Read the model definition and answer for the solid it produces. Units are mm, in the model's axes. A direction names the side the tool comes from. Coordinates: 2 decimals unless noted, no trailing zeros. Write each loop counter-clockwise with the first axis right and the second up, starting at its lowest first coordinate (ties: lowest second). Pieces come first, ordered by that corner, then holes. Notation, with made-up numbers: (34, -26.75) -> (74, -26.75) arc R31 cw to (74, 3.25) -> close; hole circle Ø4 at (53, 39.5). An arc over 180 degrees is marked (long way). One line per item, written item: value. Start each with the question number.
1. Consider line 1 along Y through (x, z) = (0, 84); line 2 along Y through (x, z) = (0, -73); line 3 along Z through (x, y) = (-60, 67). Determine where each line is inside the solid, lowest interval first.
2. Find section A-A, the plane z = 72. State how many separate pieces and enclosed holes the cut face has, and give its area (3 significant figures).
3. For a pull along Z with two mould halves and no side action, classify faces 1 (the flat face through (-22.57, 50.35, -89)), 2 (the flat face through (-25, 21, -59)), 3 (the cylindrical face through (20.59, -92.74, -79.14)) as pulls with the +Z half, pulls with the -Z half, needs draft (parallel to the pull), parting line crosses it, or undercut.
4. Find section D-D, the plane y = -83.5. Write down the section's boundary in (x, z).
5. Given P1, Ø3, axis at x = 26.5, y = 27, coming from the +Z side; P2, Ø1, axis at x = -23, y = 46.5, coming from the -Z side; P3, Ø2, axis at x = -11.5, z = -52, coming from the +Y side, each flat-ended and moving along its own axis, determine where each tip first touches the part or whether it passes through.
6. Find section B-B, the plane z = -77. Write down the section's boundary in (x, y).
7. For faces 4 (the cylindrical face through (9.764, 74.362, -79.14)), 5 (the flat face through (-24, -93, -89)), 6 (the flat face through (-1, -65, 1)), 7 (the cylindrical face through (48.627, 22.202, 68.126)), determine the directions among +Z, -Z, +X, -X, +Y, -Y from which every point of the face is accessible in a straight line to the end or side of a thin tool.
```python
from build123d import *

# Parameters (mm, degrees)
SKETCH_1_R           = 105
EXTRUDE_1_DEPTH      = 89
CUT_EXTRUDE_1_DEPTH  = 59
SKETCH_4_R           = 95
SKETCH_4_R_2         = 75
CUT_EXTRUDE_2_DEPTH  = 20
SKETCH_5_R           = 55
CUT_EXTRUDE_3_DEPTH  = 22
SKETCH_6_R           = 50
CUT_EXTRUDE_4_DEPTH  = 3
CUT_EXTRUDE_5_REACH  = 215.211
SKETCH_7_R           = 31
CUT_EXTRUDE_START    = -20
SKETCH_8_R           = 95
SKETCH_8_R_2         = 75
CUT_EXTRUDE_6_DEPTH  = 20
SKETCH_9_R           = 67.5
CUT_EXTRUDE_7_DEPTH  = 12
CUT_EXTRUDE_8_REACH  = 224.724
SKETCH_10_R          = 32.5
CHAMFER_1_SIZE       = 2
CUT_EXTRUDE_9_REACH  = 218.827
SKETCH_11_R          = 5
CUT_EXTRUDE_10_REACH = 224.724
SKETCH_12_R          = 4.5


with BuildPart() as part:
    # 草图1 → 凸台-拉伸1 (new, symmetric)
    with BuildSketch(Plane.XY):
        Circle(SKETCH_1_R)
    extrude(amount=EXTRUDE_1_DEPTH, both=True)

    # 草图3 → 切除-拉伸1 (cut, symmetric)
    with BuildSketch(Plane.XY):
        with BuildLine():
            Line((-82.462112512, -65), (82.462112512, -65))
            ThreePointArc((82.462112512, -65), (0, 105), (-82.462112512, -65))
        make_face()
    extrude(amount=CUT_EXTRUDE_1_DEPTH, both=True, mode=Mode.SUBTRACT)

    # 草图4 → 切除-拉伸2 (cut)
    with BuildSketch(Plane(origin=(0, 0, -89), x_dir=(-1, 0, 0), z_dir=(0, 0, -1))):
        Circle(SKETCH_4_R)
        Circle(SKETCH_4_R_2, mode=Mode.SUBTRACT)
    extrude(amount=-CUT_EXTRUDE_2_DEPTH, mode=Mode.SUBTRACT)

    # 草图5 → 切除-拉伸3 (cut)
    with BuildSketch(Plane(origin=(0, 0, -89), x_dir=(-1, 0, 0), z_dir=(0, 0, -1))):
        Circle(SKETCH_5_R)
    extrude(amount=-CUT_EXTRUDE_3_DEPTH, mode=Mode.SUBTRACT)

    # 草图6 → 切除-拉伸4 (cut)
    with BuildSketch(Plane(origin=(0, 0, -67), x_dir=(-1, 0, 0), z_dir=(0, 0, -1))):
        Circle(SKETCH_6_R)
    extrude(amount=-CUT_EXTRUDE_4_DEPTH, mode=Mode.SUBTRACT)

    # 草图7 → 切除-拉伸5 (cut, up to next)
    with BuildSketch(Plane(origin=(0, 0, -64), x_dir=(-1, 0, 0), z_dir=(0, 0, -1)), mode=Mode.PRIVATE) as cut_extrude_5_sk1:
        Circle(SKETCH_7_R)
    cut_extrude_5_tool1 = extrude(cut_extrude_5_sk1.sketch, amount=-CUT_EXTRUDE_5_REACH, mode=Mode.PRIVATE) & part.part
    add(cut_extrude_5_tool1.solids().sort_by_distance((0, 0, -64))[0], mode=Mode.SUBTRACT)

    # 草图8 → 切除-拉伸6 (cut)
    with BuildSketch(Plane.XY.offset(89).offset(CUT_EXTRUDE_START)):
        with Locations(Location((0, 0, 0), (0, 0, 180))):
            Circle(SKETCH_8_R)
        with Locations(Location((0, 0, 0), (0, 0, 180))):
            Circle(SKETCH_8_R_2, mode=Mode.SUBTRACT)
    extrude(amount=CUT_EXTRUDE_6_DEPTH, mode=Mode.SUBTRACT)

    # 草图9 → 切除-拉伸7 (cut)
    with BuildSketch(Plane.XY.offset(89)):
        Circle(SKETCH_9_R)
    extrude(amount=-CUT_EXTRUDE_7_DEPTH, mode=Mode.SUBTRACT)

    # 草图10 → 切除-拉伸8 (cut, up to next)
    with BuildSketch(Plane.XY.offset(77), mode=Mode.PRIVATE) as cut_extrude_8_sk1:
        Circle(SKETCH_10_R)
    cut_extrude_8_tool1 = extrude(cut_extrude_8_sk1.sketch, amount=-CUT_EXTRUDE_8_REACH, mode=Mode.PRIVATE) & part.part
    add(cut_extrude_8_tool1.solids().sort_by_distance((0, 0, 77))[0], mode=Mode.SUBTRACT)

    # 倒角1
    chamfer_1_edges = [part.edges().sort_by_distance(p)[0] for p in [
        (-32.5, 0, 77),
    ]]
    chamfer(chamfer_1_edges, length=CHAMFER_1_SIZE)

    # 草图11 → 切除-拉伸9 (cut, up to next)
    with BuildSketch(Plane.XY.offset(69), mode=Mode.PRIVATE) as cut_extrude_9_sk1:
        with Locations((0, 85)):
            Circle(SKETCH_11_R)
    cut_extrude_9_tool1 = extrude(cut_extrude_9_sk1.sketch, amount=-CUT_EXTRUDE_9_REACH, mode=Mode.PRIVATE) & part.part
    # 草图11 → 切除-拉伸9 (cut, up to next)
    with BuildSketch(Plane.XY.offset(69), mode=Mode.PRIVATE) as cut_extrude_9_sk2:
        with Locations((32.528091751, 78.529760263)):
            Circle(SKETCH_11_R)
    cut_extrude_9_tool2 = extrude(cut_extrude_9_sk2.sketch, amount=-CUT_EXTRUDE_9_REACH, mode=Mode.PRIVATE) & part.part
    # 草图11 → 切除-拉伸9 (cut, up to next)
    with BuildSketch(Plane.XY.offset(69), mode=Mode.PRIVATE) as cut_extrude_9_sk3:
        with Locations((-32.528091751, 78.529760263)):
            Circle(SKETCH_11_R)
    cut_extrude_9_tool3 = extrude(cut_extrude_9_sk3.sketch, amount=-CUT_EXTRUDE_9_REACH, mode=Mode.PRIVATE) & part.part
    add(cut_extrude_9_tool1.solids().sort_by_distance((0, 85, 69))[0], mode=Mode.SUBTRACT)
    add(cut_extrude_9_tool2.solids().sort_by_distance((32.528092, 78.52976, 69))[0], mode=Mode.SUBTRACT)
    add(cut_extrude_9_tool3.solids().sort_by_distance((-32.528092, 78.52976, 69))[0], mode=Mode.SUBTRACT)

    # 草图12 → 切除-拉伸10 (cut, up to next)
    with BuildSketch(Plane.XY.offset(77), mode=Mode.PRIVATE) as cut_extrude_10_sk1:
        with Locations((22.004297361, 53.123073119)):
            Circle(SKETCH_12_R)
    cut_extrude_10_tool1 = extrude(cut_extrude_10_sk1.sketch, amount=-CUT_EXTRUDE_10_REACH, mode=Mode.PRIVATE) & part.part
    # 草图12 → 切除-拉伸10 (cut, up to next)
    with BuildSketch(Plane.XY.offset(77), mode=Mode.PRIVATE) as cut_extrude_10_sk2:
        with Locations((53.123073119, 22.004297361)):
            Circle(SKETCH_12_R)
    cut_extrude_10_tool2 = extrude(cut_extrude_10_sk2.sketch, amount=-CUT_EXTRUDE_10_REACH, mode=Mode.PRIVATE) & part.part
    # 草图12 → 切除-拉伸10 (cut, up to next)
    with BuildSketch(Plane.XY.offset(77), mode=Mode.PRIVATE) as cut_extrude_10_sk3:
        with Locations((53.123073119, -22.004297361)):
            Circle(SKETCH_12_R)
    cut_extrude_10_tool3 = extrude(cut_extrude_10_sk3.sketch, amount=-CUT_EXTRUDE_10_REACH, mode=Mode.PRIVATE) & part.part
    # 草图12 → 切除-拉伸10 (cut, up to next)
    with BuildSketch(Plane.XY.offset(77), mode=Mode.PRIVATE) as cut_extrude_10_sk4:
        with Locations((22.004297361, -53.123073119)):
            Circle(SKETCH_12_R)
    cut_extrude_10_tool4 = extrude(cut_extrude_10_sk4.sketch, amount=-CUT_EXTRUDE_10_REACH, mode=Mode.PRIVATE) & part.part
    # 草图12 → 切除-拉伸10 (cut, up to next)
    with BuildSketch(Plane.XY.offset(77), mode=Mode.PRIVATE) as cut_extrude_10_sk5:
        with Locations((-22.004297361, -53.123073119)):
            Circle(SKETCH_12_R)
    cut_extrude_10_tool5 = extrude(cut_extrude_10_sk5.sketch, amount=-CUT_EXTRUDE_10_REACH, mode=Mode.PRIVATE) & part.part
    # 草图12 → 切除-拉伸10 (cut, up to next)
    with BuildSketch(Plane.XY.offset(77), mode=Mode.PRIVATE) as cut_extrude_10_sk6:
        with Locations((-53.123073119, -22.004297361)):
            Circle(SKETCH_12_R)
    cut_extrude_10_tool6 = extrude(cut_extrude_10_sk6.sketch, amount=-CUT_EXTRUDE_10_REACH, mode=Mode.PRIVATE) & part.part
    # 草图12 → 切除-拉伸10 (cut, up to next)
    with BuildSketch(Plane.XY.offset(77), mode=Mode.PRIVATE) as cut_extrude_10_sk7:
        with Locations((-53.123073119, 22.004297361)):
            Circle(SKETCH_12_R)
    cut_extrude_10_tool7 = extrude(cut_extrude_10_sk7.sketch, amount=-CUT_EXTRUDE_10_REACH, mode=Mode.PRIVATE) & part.part
    # 草图12 → 切除-拉伸10 (cut, up to next)
    with BuildSketch(Plane.XY.offset(77), mode=Mode.PRIVATE) as cut_extrude_10_sk8:
        with Locations((-22.004297361, 53.123073119)):
            Circle(SKETCH_12_R)
    cut_extrude_10_tool8 = extrude(cut_extrude_10_sk8.sketch, amount=-CUT_EXTRUDE_10_REACH, mode=Mode.PRIVATE) & part.part
    add(cut_extrude_10_tool1.solids().sort_by_distance((22.004297, 53.123073, 77))[0], mode=Mode.SUBTRACT)
    add(cut_extrude_10_tool2.solids().sort_by_distance((53.123073, 22.004297, 77))[0], mode=Mode.SUBTRACT)
    add(cut_extrude_10_tool3.solids().sort_by_distance((53.123073, -22.004297, 77))[0], mode=Mode.SUBTRACT)
    add(cut_extrude_10_tool4.solids().sort_by_distance((22.004297, -53.123073, 77))[0], mode=Mode.SUBTRACT)
    add(cut_extrude_10_tool5.solids().sort_by_distance((-22.004297, -53.123073, 77))[0], mode=Mode.SUBTRACT)
    add(cut_extrude_10_tool6.solids().sort_by_distance((-53.123073, -22.004297, 77))[0], mode=Mode.SUBTRACT)
    add(cut_extrude_10_tool7.solids().sort_by_distance((-53.123073, 22.004297, 77))[0], mode=Mode.SUBTRACT)
    add(cut_extrude_10_tool8.solids().sort_by_distance((-22.004297, 53.123073, 77))[0], mode=Mode.SUBTRACT)


solid = part.part
```
Answer block:
1. line 1: y = -105 to -95, -75 to -67.5, 67.5 to 75, 95 to 105
1. line 2: y = -105 to -95, -75 to -55, 55 to 75, 95 to 105
1. line 3: z = -69 to -59, 59 to 69
2. separate pieces: 2
2. enclosed holes: 10
2. area: 20,100 mm2
3. face 1: pulls with the -Z half
3. face 2: undercut
3. face 3: needs draft
4. outline: (-63.66, -89) -> (-45.31, -89) -> (-45.31, -69) -> (45.31, -69) -> (45.31, -89) -> (63.66, -89) -> (63.66, 89) -> (45.31, 89) -> (45.31, 69) -> (-45.31, 69) -> (-45.31, 89) -> (-63.66, 89) -> close
5. P1: stops at z = 77
5. P2: stops at z = -67
5. P3: stops at y = -65
6. outline: circle Ø210 at (0, 0); circle Ø150 at (0, 0); hole circle Ø190 at (0, 0); hole circle Ø110 at (0, 0)
7. face 4: -Z
7. face 5: -Z, +X, -X, +Y, -Y
7. face 6: +X, -X, +Y
7. face 7: +Z
